Work out the finished part from the listing and answer in its coordinate system (mm). Coordinates: 2 decimals unless noted, no trailing zeros. Write each loop counter-clockwise with the first axis right and the second up, starting at its lowest first coordinate (ties: lowest second). Pieces come first, ordered by that corner, then holes. Notation, with made-up numbers: M 53.5,12.5 L 104.5,12.5 A32 cw 104.5,49.5 Z; hole C 21,-8 d10. An arc over 180 degrees is marked long. Answer as CSV lines item,"result". Start each with the question number.
(1) A cutting plane is placed at D-D on x = 27.5. Give the vertices of the cut face in (y, z), then the cut area to 3 significant figures.
(2) A cutting plane is placed at A-A on x = 0. Give the vertices of the cut face in (y, z).
(3) A cutting plane is placed at C-C on y = -65. Give the vertices of the cut face in (x, z).
(4) Find the intervals of material crossed by L1, parallel to X at y = -65, z = 1.45; L2, parallel to Y at x = 9, z = 4.4; L3, parallel to X at y = -71, z = 3.9, in increasing order. Write a range as [from, to].
(5) The mould has two halves that part along Y. Classify faces 1 (the flat face through (-1, -1.5, 2)), 2 (the flat face through (29.228, -43.925, 2.465)), 3 (the cylindrical face through (1.627, -77.394, 2.465)), 4 (the flat face through (1, -33, 0)): released by +Y, released by -Y, zero draft, split by the parting line, or undercut.
(6) A cutting plane is placed at B-B on z = 2.35. Give the vertices of the cut face in (x, y).
from build123d import *

# Parameters (mm, degrees)
SKETCH_2_R             = 12.5
SM_BASE_FLANGE_1_DEPTH = 5


# Sheet-metal steps are written as plain solids
with BuildPart() as part:
    # Sketch 2 → Базовая кромка1 (new body)
    with BuildSketch(Plane.XY):
        with BuildLine():
            Line((-18.150140865, -72.128982157), (-40, -16.5))
            Line((-40, -16.5), (-40, -1.5))
            Line((-40, -1.5), (40, -1.5))
            Line((40, -1.5), (40, -16.5))
            Line((40, -16.5), (18.150140865, -72.128982157))
            ThreePointArc((18.150140865, -72.128982157), (0, -84.5), (-18.150140865, -72.128982157))
        make_face()
        with Locations(Location((0, -65, 0), (0, 0, 180))):
            Circle(SKETCH_2_R, mode=Mode.SUBTRACT)
    extrude(amount=SM_BASE_FLANGE_1_DEPTH)


solid = part.part
Here are the results:
1,outline,"M -48.32,0 L -1.5,0 L -1.5,5 L -48.32,5 Z"
1,area,"234 mm^2"
2,outline,"M -84.5,0 L -77.5,0 L -77.5,5 L -84.5,5 Z; M -52.5,0 L -1.5,0 L -1.5,5 L -52.5,5 Z"
3,outline,"M -20.95,0 L -12.5,0 L -12.5,5 L -20.95,5 Z; M 12.5,0 L 20.95,0 L 20.95,5 L 12.5,5 Z"
4,L1,"x = [-20.95, -12.5], [12.5, 20.95]"
4,L2,"y = [-82.3, -73.67], [-56.33, -1.5]"
4,L3,"x = [-18.59, -10.97], [10.97, 18.59]"
5,face 1,"released by +Y"
5,face 2,"released by -Y"
5,face 3,"undercut"
5,face 4,"zero draft"
6,outline,"M -40,-16.5 L -18.15,-72.13 A19.5 ccw 18.15,-72.13 L 40,-16.5 L 40,-1.5 L -40,-1.5 Z; hole C 0,-65 d25"
